The drawing under review shows one solid part. Ordinate dimensions are in mm from its lowest x, y, z. A direction names the side the tool comes from. Coordinates: 2 decimals unless noted, no trailing zeros. Order: outer loops, then holes, each group sorted by start corner. A loop starts at its lowest first (then second) coordinate and runs counter-clockwise, first axis right, second up.
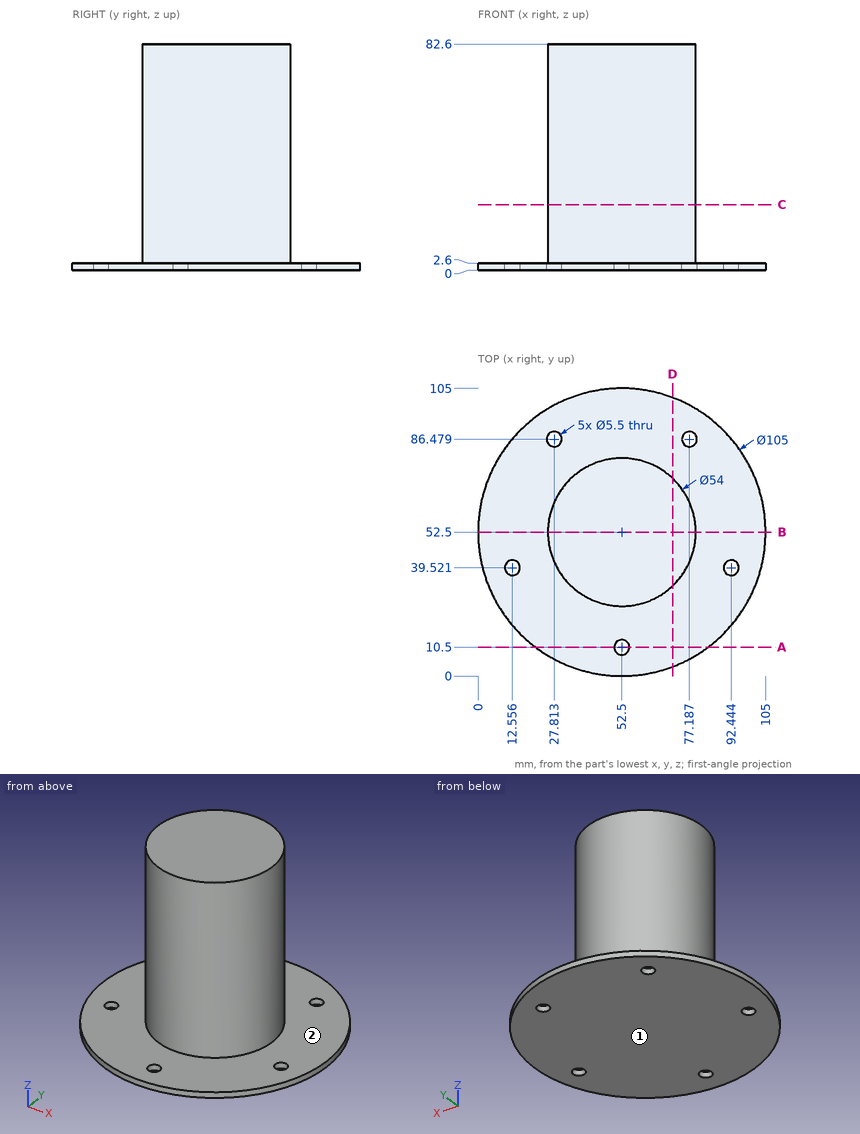
(1) Machinability: for the marked faces 1 and 2, which of the approach directions +Z, -Z, +X, -X, +Y, -Y give a long, thin tool a straight path to every point of the face, cutting with its end or side? Answer none if there is none.
A:
face 1: -Z, +X, -X, +Y, -Y
face 2: +Z
(2) Wall thickness on probe 1 along Z at (x, y) = (19, 36); probe 2 along Y at (x, z) = (52.5, 1.5); probe 3 along Y at (x, z) = (61.5, 74) (1 decimal): over which ranges is each line inside the solid? List them lowest first.
A:
probe 1: z = 0 to 2.6
probe 2: y = 0 to 7.75, 13.25 to 105
probe 3: y = 27 to 78
(3) For pin 1 Ø8 at (y, z) = (52.5, 38.5) entering from -X; pin 2 Ø4.5 at (x, y) = (92.44, 39.52) entering from -Z; pin 3 Ø5 at (y, z) = (71, 54.5) entering from -X; pin 4 Ø2 at (x, y) = (41.5, 24.5) entering from +Z, all flat-tipped, find the tip position at first contact; note any pin that passes through.
A:
pin 1: stops at x = 25.5
pin 2: passes through
pin 3: stops at x = 30.75
pin 4: stops at z = 2.6
(4) We need section D-D, the plane x = 71. Write out the cut boundary in (y, z), and give its area (3 significant figures).
A:
outline: (3.37, 0) - (101.63, 0) - (101.63, 2.6) - (72.17, 2.6) - (72.17, 82.6) - (32.83, 82.6) - (32.83, 2.6) - (3.37, 2.6) - close
area: 3,400 mm2
(5) We need section C-C, the plane z = 24. Write out the cut boundary in (x, y), and give its area (3 significant figures).
A:
outline: circle Ø54 at (52.5, 52.5)
area: 2,290 mm2
(6) We need section A-A, the plane y = 10.5. Write out the cut boundary in (x, z).
A:
outline: (21, 0) - (49.75, 0) - (49.75, 2.6) - (21, 2.6) - close; (55.25, 0) - (84, 0) - (84, 2.6) - (55.25, 2.6) - close
(7) We need section B-B, the plane y = 52.5. Write out the cut boundary in (x, z).
A:
outline: (0, 0) - (105, 0) - (105, 2.6) - (79.5, 2.6) - (79.5, 82.6) - (25.5, 82.6) - (25.5, 2.6) - (0, 2.6) - close
